```python
from build123d import *

# Parameters (mm, degrees)
SKETCH1_W                = 25
SKETCH1_H                = 24
BOSS_EXTRUDE1_DEPTH      = 1
SKETCH2_R                = 1
SKETCH2_R_2              = 0.75
CUT_EXTRUDE1_DEPTH       = 2
SKETCH3_R                = 2
SKETCH3_R_2              = 1
BOSS_EXTRUDE3_DEPTH      = 0.1
BOSS_EXTRUDE3_DEPTH_BACK = 1.1
SKETCH4_W                = 1.7
SKETCH4_H                = 2.5
BOSS_EXTRUDE4_DEPTH      = 1
FILLET1_R                = 0.1
SKETCH5_W                = 2
SKETCH5_H                = 1
SKETCH5_H_2              = 1.5
BOSS_EXTRUDE5_DEPTH      = 0.5


with BuildPart() as part:
    # Sketch1 → Boss-Extrude1 (new body)
    with BuildSketch(Plane.XY):
        Rectangle(SKETCH1_W, SKETCH1_H)
    extrude(amount=BOSS_EXTRUDE1_DEPTH)

    # Sketch2 → Cut-Extrude1 (cut)
    with BuildSketch(Plane.XY.offset(1)):
        with Locations((-10.5, 10)):
            Circle(SKETCH2_R)
        with Locations((10.5, 10)):
            Circle(SKETCH2_R)
        with Locations((10.5, -4)):
            Circle(SKETCH2_R)
        with Locations((-10.5, -4)):
            Circle(SKETCH2_R)
        with Locations((-9, 3)):
            Circle(SKETCH2_R_2)
        with Locations((9, 3)):
            Circle(SKETCH2_R_2)
    extrude(amount=-CUT_EXTRUDE1_DEPTH, mode=Mode.SUBTRACT)

    # Sketch3 → Boss-Extrude3 (add, two sides)
    with BuildSketch(Plane.XY.offset(1)) as boss_extrude3_sk:
        with Locations((-10.5, 10)):
            Circle(SKETCH3_R)
        with Locations((-10.5, 10)):
            Circle(SKETCH3_R_2, mode=Mode.SUBTRACT)
        with Locations((10.5, 10)):
            Circle(SKETCH3_R)
        with Locations((10.5, 10)):
            Circle(SKETCH3_R_2, mode=Mode.SUBTRACT)
        with Locations((10.5, -4)):
            Circle(SKETCH3_R)
        with Locations((10.5, -4)):
            Circle(SKETCH3_R_2, mode=Mode.SUBTRACT)
        with Locations((-10.5, -4)):
            Circle(SKETCH3_R)
        with Locations((-10.5, -4)):
            Circle(SKETCH3_R_2, mode=Mode.SUBTRACT)
    extrude(amount=BOSS_EXTRUDE3_DEPTH)
    extrude(boss_extrude3_sk.sketch, amount=-BOSS_EXTRUDE3_DEPTH_BACK)

    # Sketch4 → Boss-Extrude4 (add)
    with BuildSketch(Plane.XY.offset(1)):
        with Locations((7.65, 6.75)):
            Rectangle(SKETCH4_W, SKETCH4_H)
    extrude(amount=BOSS_EXTRUDE4_DEPTH)

    # Fillet1
    fillet1_edges = [part.edges().sort_by_distance(p)[0] for p in [
        (8.5, 6.75, 2),
        (7.65, 8, 2),
        (6.8, 6.75, 2),
        (7.65, 5.5, 2),
    ]]
    fillet(fillet1_edges, radius=FILLET1_R)

    # Sketch5 → Boss-Extrude5 (add)
    with BuildSketch(Plane.XY.offset(1)):
        with Locations((-8, 0)):
            Rectangle(SKETCH5_W, SKETCH5_H)
        with Locations((8, -0.25)):
            Rectangle(SKETCH5_W, SKETCH5_H_2)
    extrude(amount=BOSS_EXTRUDE5_DEPTH)


solid = part.part
```
Check sheet for the modelled part. Datum: model origin and axes. Units: mm. A direction names the side the tool comes from. Round coordinates to 2 decimals unless told otherwise and drop trailing zeros. Order: outer loops, then holes, each group sorted by start corner. A loop starts at its lowest first (then second) coordinate and runs counter-clockwise, first axis right, second up.
1) Scan lines: line 1 (Y direction, x = 10.5, z = 0.05); line 2 (Z direction, x = -5, y = 10); line 3 (Z direction, x = -11.25, y = 10.75). Record each from-to range of solid material in increasing order.
2) Section check A-A (x = -6). Record the boundary of the cut face in (y, z), and give its area (3 significant figures).
3) Go/stop test with flat-tipped pins: pin 1 Ø3 at (x, y) = (-10.5, -4) entering from +Z; pin 2 Ø4 at (x, y) = (5.5, -7.5) entering from -Z; pin 3 Ø3 at (x, y) = (2.5, -3) entering from +Z. Record where each tip stops, or that it passes through.
4) Section check B-B (y = 1.5). Record the boundary of the cut face in (x, z).
5) Mould release check, pull along Z, two halves, no side actions. Record for faces 4 (the flat face through (7.6, 8, 1.4)), 5 (the flat face through (11.4, 9.1, 1.1)), 6 (the flat face through (-9.6, 9.1, -0.1)): +Z half, -Z half, draft (parallel to the pull), parting line (faces both ways), or undercut.
6) Tool access check on faces 1 (the flat face through (-12.1, 11.5, 0)), 2 (the flat face through (-0.2, -12, 0.5)), 3 (the flat face through (8, 0, 1.5)). Record the directions out of +Z, -Z, +X, -X, +Y, -Y that give a thin tool (end or side, any length) a straight path to the whole face; none if there is none.
Result:
1. line 1: y = -12 to -5, -3 to 9, 11 to 12
1. line 2: z = 0 to 1
1. line 3: z = -0.1 to 1.1
2. outline: (-12, 0) - (12, 0) - (12, 1) - (-12, 1) - close
2. area: 24.0 mm2
3. pin 1: stops at z = 1.1
3. pin 2: stops at z = 0
3. pin 3: stops at z = 1
4. outline: (-12.5, 0) - (12.5, 0) - (12.5, 1) - (-12.5, 1) - close
5. face 4: draft
5. face 5: +Z half
5. face 6: -Z half
6. face 1: -Z, -X, +Y
6. face 2: +Z, -Z, +X, -X, -Y
6. face 3: +Z, +X, -X, -Y
